The figure shows three views and two pictorial views of one solid part (mm, origin at its lowest corner). Answer the questions. A direction names the side the tool comes from. Round coordinates to 2 decimals unless told otherwise and drop trailing zeros. Order: outer loops, then holes, each group sorted by start corner. A loop starts at its lowest first (then second) coordinate and runs counter-clockwise, first axis right, second up. Notation, with made-up numbers: (77.5, 64.25) - (107.5, 64.25) arc R26 ccw to (107.5, 96.25) - close; hole circle Ø5 at (-8.75, 4). An arc over 180 degrees is marked (long way). One line per item, written item: value. Start each with the question number.
1. For a pull along Y with two mould halves and no side action, classify the marked faces 1, 2 and 3 as released by +Y, released by -Y, zero draft, split by the parting line, or undercut.
2. Straight lines are drawn through the part: line 1 (Y direction, x = 10.5, z = 5.75) (1 decimal); line 2 (Y direction, x = 9.75, z = 9.25) (1 decimal); line 3 (X direction, y = 11.25, z = 5.25) (1 decimal). For each, find the intervals that lie inside material, in ascending order.
3. Section A-A, the plane z = 9.25 is taken. Give the vertices of the cut face in (x, y) (1 decimal).
4. Section D-D, the plane x = 7.5 is taken. Give the vertices of the cut face in (y, z) (1 decimal).
5. Section B-B, the plane y = 9 is taken. Give the vertices of the cut face in (x, z) (1 decimal), then the cut area to 3 significant figures.
6. Flat-ended cylindrical pins translate along their axes: P1, Ø4, axis at x = 1, z = 4.5, coming from the +Y side; P2, Ø5.5, axis at y = 8.5, z = 4.5, coming from the +X side; P3, Ø1.5, axis at y = 8, z = 5.5, coming from the -X side. Find the tip coordinate at first contact, or state that the pin passes through.
7. Section C-C, the plane x = 5.5 is taken. Give the vertices of the cut face in (y, z).
8. A tool of negligible diameter and unlimited length cuts with its end or side. For the marked faces 4, 5, 6, 7 and 8, from which of +Z, -Z, +X, -X, +Y, -Y can it reach the whole face along a straight path? Write none if from no direction.
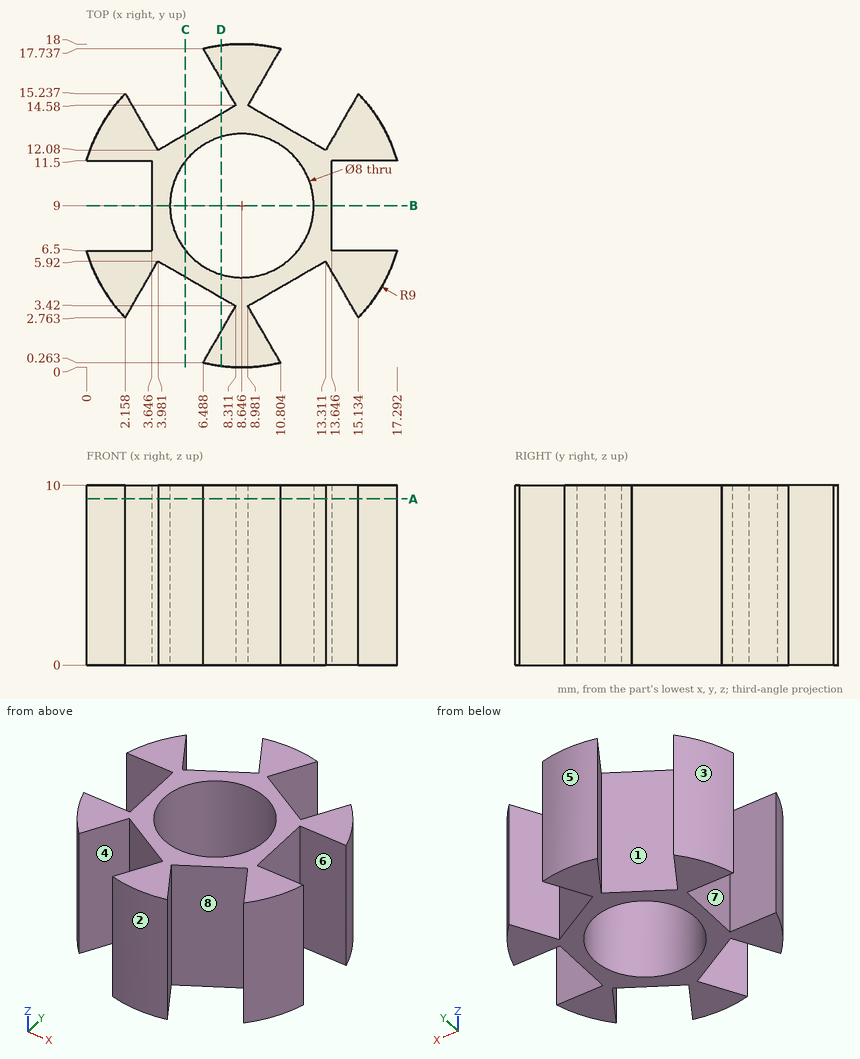
Answer list:
1. face 1: undercut
1. face 2: released by -Y
1. face 3: released by +Y
2. line 1: y = 0.2 to 0.8, 4.3 to 5.5, 12.5 to 13.7, 17.2 to 17.8
2. line 2: y = 0.1 to 2.1, 3.9 to 5.2, 12.8 to 14.1, 15.9 to 17.9
2. line 3: x = 3.6 to 5.3, 12 to 13.6
3. outline: (0, 6.5) arc R9 ccw to (2.2, 2.8) - (4, 5.9) - (8.3, 3.4) - (6.5, 0.3) arc R9 ccw to (10.8, 0.3) - (9, 3.4) - (13.3, 5.9) - (15.1, 2.8) arc R9 ccw to (17.3, 6.5) - (13.6, 6.5) - (13.6, 11.5) - (17.3, 11.5) arc R9 ccw to (15.1, 15.2) - (13.3, 12.1) - (9, 14.6) - (10.8, 17.7) arc R9 ccw to (6.5, 17.7) - (8.3, 14.6) - (4, 12.1) - (2.2, 15.2) arc R9 ccw to (0, 11.5) - (3.6, 11.5) - (3.6, 6.5) - close; hole circle Ø8 at (8.6, 9)
4. outline: (0.1, 0) - (2, 0) - (2, 10) - (0.1, 10) - close; (3.9, 0) - (5.2, 0) - (5.2, 10) - (3.9, 10) - close; (12.8, 0) - (14.1, 0) - (14.1, 10) - (12.8, 10) - close; (16, 0) - (17.9, 0) - (17.9, 10) - (16, 10) - close
5. outline: (3.6, 0) - (4.6, 0) - (4.6, 10) - (3.6, 10) - close; (12.6, 0) - (13.6, 0) - (13.6, 10) - (12.6, 10) - close
5. area: 20.0 mm²
6. P1: stops at y = 15.24
6. P2: stops at x = 17.29
6. P3: stops at x = 3.65
7. outline: (5.04, 0) - (6.53, 0) - (6.53, 10) - (5.04, 10) - close; (11.47, 0) - (12.96, 0) - (12.96, 10) - (11.47, 10) - close
8. face 4: +Z, -Z, -Y
8. face 5: +Z, -Z, +Y
8. face 6: +Z, -Z, +X
8. face 7: +Z, -Z, -X
8. face 8: +Z, -Z
